Can you work these out from the model? Positions are in its coordinate system, mm. Face numbers are marked on the shaded views. A direction names the side the tool comes from. Round coordinates to 2 decimals unless told otherwise and drop trailing zeros. Write each loop counter-clockwise with the first axis right and the second up, starting at its lowest first coordinate (ties: lowest second). Pieces come first, ordered by that corner, then holes. Notation, with made-up numbers: (9.25, 62) -> (42.25, 62) arc R32 ccw to (42.25, 94) -> close; hole circle Ø7 at (67.25, 21.25). An arc over 180 degrees is marked (long way). Use CSV: the item, a comma, the result in double quotes.
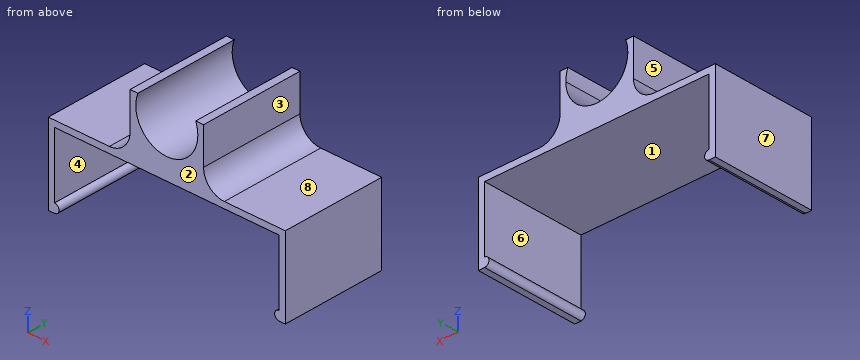
```python
from build123d import *

# Parameters (mm, degrees)
F1_DEPTH = 12.7
F3_DEPTH = 25.4
F5_W     = 18
F5_H     = 25.4
F6_DEPTH = 14
F8_DEPTH = 25.401
F9_R     = 5.08


with BuildPart() as f1:
    # F0 (on Front) → F1 (new body, symmetric)
    with BuildSketch(Plane.XZ):
        Polygon((27.5, 18), (27.5, 0), (29.024, 0), (29.024, 19.524), (0, 19.524), (-29.024, 19.524), (-29.024, 0), (-27.5, 0), (-27.5, 18), (0, 18), align=None)
    extrude(amount=F1_DEPTH, both=True)

    # F2 (on face) → F3 (join, through all)
    with BuildSketch(Plane.XZ.offset(12.7)):
        with BuildLine():
            Line((-27.5, 2.1935291588), (-27.5, 0))
            ThreePointArc((-27.5, 0), (-26.4032354206, 1.0967645794), (-27.5, 2.1935291588))
        make_face()
    extrude(amount=-F3_DEPTH)

    # F4: F1 across plane


with BuildPart() as f1_1:
    add(f1.part)
    add(f1.part.mirror(Plane.YZ))

    # F5 (on face) → F6 (join)
    with BuildSketch(Plane.XY.offset(19.524)):
        Rectangle(F5_W, F5_H)
    extrude(amount=F6_DEPTH)

    # F7 (on face) → F8 (cut, through all)
    with BuildSketch(Plane.XZ.offset(12.7)):
        with BuildLine():
            ThreePointArc((-7.0774375942, 33.524), (-1.409161858, 23.2863288576), (7.6, 30.7545457035))
            ThreePointArc((7.6, 30.7545457035), (7.4682168459, 32.1637075615), (7.0774375942, 33.524))
            Line((7.0774375942, 33.524), (-7.0774375942, 33.524))
        make_face()
    extrude(amount=-F8_DEPTH, mode=Mode.SUBTRACT)

    # F9
    f9_edges = [f1_1.edges().sort_by_distance(p)[0] for p in [
        (9, 0, 19.524),
        (-9, 0, 19.524),
    ]]
    fillet(f9_edges, radius=F9_R)


solid = f1_1.part
```
Q1. Will these pins go through, and if not, where does the flat tip stop? P1, Ø12, axis at x = -24.5, y = -5.5, coming from the +Z side; P2, Ø7.5, axis at x = -2, y = -4, coming from the -Z side; P3, Ø10, axis at y = -4, z = 28, coming from the +X side.
Resolved:
P1,"stops at z = 19.52"
P2,"stops at z = 18"
P3,"stops at x = 9.26"
Q2. Suppose I cut it at B-B (y = 5.5). Write out the boundary of the cut face in (x, z), and give its area (3 significant figures).
Resolved:
outline,"(-29.02, 0) -> (-27.5, 0) arc R1.1 ccw to (-27.5, 2.19) -> (-27.5, 18) -> (27.5, 18) -> (27.5, 2.19) arc R1.1 ccw to (27.5, 0) -> (29.02, 0) -> (29.02, 19.52) -> (14.08, 19.52) arc R5.08 cw to (9, 24.6) -> (9, 33.52) -> (7.08, 33.52) arc R7.6 cw (long way) to (-7.08, 33.52) -> (-9, 33.52) -> (-9, 24.6) arc R5.08 cw to (-14.08, 19.52) -> (-29.02, 19.52) -> close"
area,"278 mm^2"
Q3. If we mould it in two halves opening along X, with no side actions, what happens to the marked faces 1, 2, 3 and 4? For each: released by +X, released by -X, zero draft, split by the parting line, or undercut.
Resolved:
face 1,"undercut"
face 2,"zero draft"
face 3,"released by +X"
face 4,"undercut"
Q4. Suppose I cut it at C-C (x = -23). Write out the boundary of the cut face in (y, z), and give its area (3 significant figures).
Resolved:
outline,"(-12.7, 18) -> (12.7, 18) -> (12.7, 19.52) -> (-12.7, 19.52) -> close"
area,"38.7 mm^2"
Q5. Suppose I cut it at A-A (z = 28). Write out the boundary of the cut face in (x, y), and give its area (3 significant figures).
Resolved:
outline,"(-9, -12.7) -> (-7.08, -12.7) -> (-7.08, 12.7) -> (-9, 12.7) -> close; (7.08, -12.7) -> (9, -12.7) -> (9, 12.7) -> (7.08, 12.7) -> close"
area,"97.4 mm^2"
Q6. Suppose I cut it at D-D (z = 7.5). Write out the boundary of the cut face in (x, y), and give its area (3 significant figures).
Resolved:
outline,"(-29.02, -12.7) -> (-27.5, -12.7) -> (-27.5, 12.7) -> (-29.02, 12.7) -> close; (27.5, -12.7) -> (29.02, -12.7) -> (29.02, 12.7) -> (27.5, 12.7) -> close"
area,"77.4 mm^2"
Q7. Please list where these lines run through material, in increasing order: probe 1 along X at (y, z) = (-1, 2.5); probe 2 along Z at (x, y) = (14, -8.25); probe 3 along X at (y, z) = (11.75, 32.5).
Resolved:
probe 1,"x = -29.02 to -27.5, 27.5 to 29.02"
probe 2,"z = 18 to 19.52"
probe 3,"x = -9 to -7.4, 7.4 to 9"
Q8. On a 3-axis mill with a long thin cutter (end or side, diameter ignored), from which of +Z, -Z, +X, -X, +Y, -Y can I reach the whole of each face in a straight line? I mean the marked faces 5, 6, 7 and 8. Say none if no direction works.
Resolved:
face 5,"+Z, -X, +Y, -Y"
face 6,"+Y, -Y"
face 7,"+Z, -Z, -X, +Y, -Y"
face 8,"+Z, +X, +Y, -Y"
